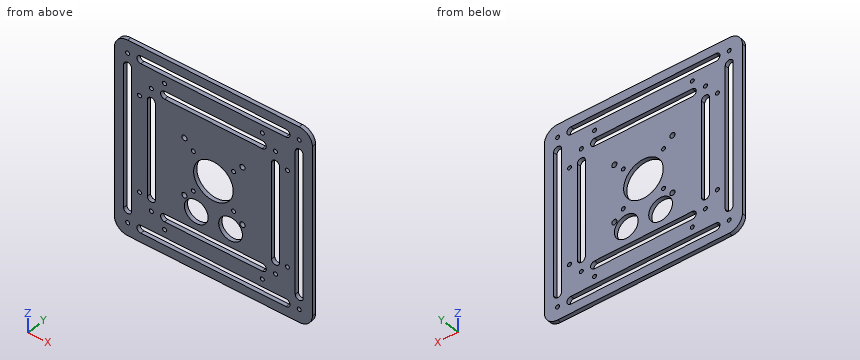
from build123d import *

# Parameters (mm, degrees)
SKETCH1_R           = 1.5
SKETCH1_R_2         = 15
SKETCH1_R_3         = 9
SKETCH1_R_4         = 2
BOSS_EXTRUDE1_DEPTH = 3


with BuildPart() as part:
    # Sketch1 → Boss-Extrude1 (new body)
    with BuildSketch(Plane(origin=(0, 0, 0), x_dir=(1, 0, 0), z_dir=(0, 1, 0))):
        with BuildLine():
            Line((-65, -75), (65, -75))
            ThreePointArc((65, -75), (72.071067812, -72.071067812), (75, -65))
            Line((75, -65), (75, 65))
            ThreePointArc((75, 65), (72.071067812, 72.071067812), (65, 75))
            Line((65, 75), (-65, 75))
            ThreePointArc((-65, 75), (-72.071067812, 72.071067812), (-75, 65))
            Line((-75, 65), (-75, -65))
            ThreePointArc((-75, -65), (-72.071067812, -72.071067812), (-65, -75))
        make_face()
        with Locations(Location((65, 65, 0), (0, 0, 270))):
            Circle(SKETCH1_R, mode=Mode.SUBTRACT)
        with Locations(Location((47.039487758, 47.039487758, 0), (0, 0, 270))):
            Circle(SKETCH1_R, mode=Mode.SUBTRACT)
        with Locations(Location((-65, 65, 0), (0, 0, 90))):
            Circle(SKETCH1_R, mode=Mode.SUBTRACT)
        with Locations(Location((-47.039487758, 47.039487758, 0), (0, 0, 90))):
            Circle(SKETCH1_R, mode=Mode.SUBTRACT)
        with Locations(Location((65, -65, 0), (0, 0, 90))):
            Circle(SKETCH1_R, mode=Mode.SUBTRACT)
        with Locations(Location((47.039487758, -47.039487758, 0), (0, 0, 90))):
            Circle(SKETCH1_R, mode=Mode.SUBTRACT)
        with Locations(Location((-65, -65, 0), (0, 0, 270))):
            Circle(SKETCH1_R, mode=Mode.SUBTRACT)
        with Locations(Location((-47.039487758, -47.039487758, 0), (0, 0, 270))):
            Circle(SKETCH1_R, mode=Mode.SUBTRACT)
        with Locations(Location((0, 0, 0), (0, 0, 270))):
            Circle(SKETCH1_R_2, mode=Mode.SUBTRACT)
        with Locations(Location((-56.039487758, 37.039487758, 0), (0, 0, 270))):
            Circle(SKETCH1_R, mode=Mode.SUBTRACT)
        with Locations(Location((-56.039487758, -37.039487758, 0), (0, 0, 90))):
            Circle(SKETCH1_R, mode=Mode.SUBTRACT)
        with Locations(Location((56.039487758, -37.039487758, 0), (0, 0, 270))):
            Circle(SKETCH1_R, mode=Mode.SUBTRACT)
        with Locations(Location((56.039487758, 37.039487758, 0), (0, 0, 90))):
            Circle(SKETCH1_R, mode=Mode.SUBTRACT)
        with Locations(Location((-37.039487758, 56.039487758, 0), (0, 0, 90))):
            Circle(SKETCH1_R, mode=Mode.SUBTRACT)
        with Locations(Location((37.039487758, 56.039487758, 0), (0, 0, 270))):
            Circle(SKETCH1_R, mode=Mode.SUBTRACT)
        with Locations(Location((-37.039487758, -56.039487758, 0), (0, 0, 270))):
            Circle(SKETCH1_R, mode=Mode.SUBTRACT)
        with Locations(Location((37.039487758, -56.039487758, 0), (0, 0, 90))):
            Circle(SKETCH1_R, mode=Mode.SUBTRACT)
        with Locations(Location((-15.25, 15.25, 0), (0, 0, 270))):
            Circle(SKETCH1_R, mode=Mode.SUBTRACT)
        with Locations(Location((15.25, 15.25, 0), (0, 0, 90))):
            Circle(SKETCH1_R, mode=Mode.SUBTRACT)
        with Locations(Location((-15.25, -15.25, 0), (0, 0, 90))):
            Circle(SKETCH1_R, mode=Mode.SUBTRACT)
        with Locations(Location((15.25, -15.25, 0), (0, 0, 90))):
            Circle(SKETCH1_R, mode=Mode.SUBTRACT)
        with Locations(Location((-13, 30.039487758, 0), (0, 0, 270))):
            Circle(SKETCH1_R_3, mode=Mode.SUBTRACT)
        with Locations(Location((13, 30.039487758, 0), (0, 0, 90))):
            Circle(SKETCH1_R_3, mode=Mode.SUBTRACT)
        with Locations(Location((-22, 22, 0), (0, 0, 270))):
            Circle(SKETCH1_R_4, mode=Mode.SUBTRACT)
        with Locations(Location((22, 22, 0), (0, 0, 90))):
            Circle(SKETCH1_R_4, mode=Mode.SUBTRACT)
        with Locations(Location((22, -22, 0), (0, 0, 90))):
            Circle(SKETCH1_R_4, mode=Mode.SUBTRACT)
        with Locations(Location((-22, -22, 0), (0, 0, 90))):
            Circle(SKETCH1_R_4, mode=Mode.SUBTRACT)
        with BuildLine():
            Line((-44.039487758, 37.039487758), (-44.039487758, -37.039487758))
            ThreePointArc((-44.039487758, -37.039487758), (-47.039487758, -40.039487758), (-50.039487758, -37.039487758))
            Line((-50.039487758, -37.039487758), (-50.039487758, 37.039487758))
            ThreePointArc((-50.039487758, 37.039487758), (-47.039487758, 40.039487758), (-44.039487758, 37.039487758))
        make_face(mode=Mode.SUBTRACT)
        with BuildLine():
            Line((44.039487758, 37.039487758), (44.039487758, -37.039487758))
            ThreePointArc((44.039487758, -37.039487758), (47.039487758, -40.039487758), (50.039487758, -37.039487758))
            Line((50.039487758, -37.039487758), (50.039487758, 37.039487758))
            ThreePointArc((50.039487758, 37.039487758), (47.039487758, 40.039487758), (44.039487758, 37.039487758))
        make_face(mode=Mode.SUBTRACT)
        with BuildLine():
            Line((-37.039487758, 44.039487758), (37.039487758, 44.039487758))
            ThreePointArc((37.039487758, 44.039487758), (40.039487758, 47.039487758), (37.039487758, 50.039487758))
            Line((37.039487758, 50.039487758), (-37.039487758, 50.039487758))
            ThreePointArc((-37.039487758, 50.039487758), (-40.039487758, 47.039487758), (-37.039487758, 44.039487758))
        make_face(mode=Mode.SUBTRACT)
        with BuildLine():
            Line((37.039487758, -44.039487758), (-37.039487758, -44.039487758))
            ThreePointArc((-37.039487758, -44.039487758), (-40.039487758, -47.039487758), (-37.039487758, -50.039487758))
            Line((-37.039487758, -50.039487758), (37.039487758, -50.039487758))
            ThreePointArc((37.039487758, -50.039487758), (40.039487758, -47.039487758), (37.039487758, -44.039487758))
        make_face(mode=Mode.SUBTRACT)
        with BuildLine():
            Line((-62, 55), (-62, -55))
            ThreePointArc((-62, -55), (-65, -58), (-68, -55))
            Line((-68, -55), (-68, 55))
            ThreePointArc((-68, 55), (-65, 58), (-62, 55))
        make_face(mode=Mode.SUBTRACT)
        with BuildLine():
            Line((62, 55), (62, -55))
            ThreePointArc((62, -55), (65, -58), (68, -55))
            Line((68, -55), (68, 55))
            ThreePointArc((68, 55), (65, 58), (62, 55))
        make_face(mode=Mode.SUBTRACT)
        with BuildLine():
            Line((-55, 62), (55, 62))
            ThreePointArc((55, 62), (58, 65), (55, 68))
            Line((55, 68), (-55, 68))
            ThreePointArc((-55, 68), (-58, 65), (-55, 62))
        make_face(mode=Mode.SUBTRACT)
        with BuildLine():
            Line((55, -62), (-55, -62))
            ThreePointArc((-55, -62), (-58, -65), (-55, -68))
            Line((-55, -68), (55, -68))
            ThreePointArc((55, -68), (58, -65), (55, -62))
        make_face(mode=Mode.SUBTRACT)
    extrude(amount=BOSS_EXTRUDE1_DEPTH)


solid = part.part
The model under review builds one solid part; all positions refer to its coordinate system, in mm. Round coordinates to 2 decimals unless told otherwise and drop trailing zeros. Write each loop counter-clockwise with the first axis right and the second up, starting at its lowest first coordinate (ties: lowest second). Pieces come first, ordered by that corner, then holes. Notation, with made-up numbers: M 47,10.25 L 62,10.25 A19 cw 62,31.25 Z; hole C -22.75,18 d7. An arc over 180 degrees is marked long. Use a Markdown table: item, result. Add a question column.
Q1. We need section C-C, the plane y = 1.1. Count the separate pieces of the cut face and the enclosed holes in it, plus the area to 3 significant figures.
Q2. We need section B-B, the plane z = 1. State the section outline as (x, y) points, plus the area to 3 significant figures.
Q3. To check wall thickness, follow line 1 (Z direction, x = -50.5, y = 0.95); line 2 (Z direction, x = -25, y = 2.65). State the ranges of each line that lie inside material, in increasing order.
Q4. We need section A-A, the plane z = 22. State the section outline as (x, y) points, plus the area to 3 significant figures.
Q5. Insertion check: pin 1 (14.5 mm diameter, centred on x = -13, z = -30.04, fed in from -Y). The pin has a flat end and moves straight along its axis. Give the tip position at first contact, or say it passes through.
Findings below:
| question | item | result |
|---|---|---|
| 1 | separate pieces | 1 |
| 1 | enclosed holes | 35 |
| 1 | area | 16,400 mm² |
| 2 | outline | M -75,0 L -68,0 L -68,3 L -75,3 Z; M -62,0 L -50.04,0 L -50.04,3 L -62,3 Z; M -44.04,0 L -14.97,0 L -14.97,3 L -44.04,3 Z; M 14.97,0 L 44.04,0 L 44.04,3 L 14.97,3 Z; M 50.04,0 L 62,0 L 62,3 L 50.04,3 Z; M 68,0 L 75,0 L 75,3 L 68,3 Z |
| 2 | area | 288 mm² |
| 3 | line 1 | z = -75 to -68, -62 to 62, 68 to 75 |
| 3 | line 2 | z = -75 to -68, -62 to -50.04, -44.04 to 44.04, 50.04 to 62, 68 to 75 |
| 4 | outline | M -75,0 L -68,0 L -68,3 L -75,3 Z; M -62,0 L -50.04,0 L -50.04,3 L -62,3 Z; M -44.04,0 L -24,0 L -24,3 L -44.04,3 Z; M -20,0 L 20,0 L 20,3 L -20,3 Z; M 24,0 L 44.04,0 L 44.04,3 L 24,3 Z; M 50.04,0 L 62,0 L 62,3 L 50.04,3 Z; M 68,0 L 75,0 L 75,3 L 68,3 Z |
| 4 | area | 354 mm² |
| 5 | pin 1 | passes through |
